Autodesk Inventor part; units mm, degrees
ref_plane "YZ Plane" through (0, 0, 0) normal (1, 0, 0) x (0, 1, 0)
ref_plane "XZ Plane" through (0, 0, 0) normal (0, 1, 0) x (-1, 0, 0)
ref_plane "XY Plane" through (0, 0, 0) normal (0, 0, 1) x (1, 0, 0)
sketch "Skizze1" plane through (0, 0, 0) normal (0, 0, 1) x (1, 0, 0)
  line L0 (-3.2332, 0) -> (3.2332, 0) construction
  line L1 (0, -2.8) -> (0, 2.8) construction
  circle A0 centre (0, 0) radius 2 construction
  line L2 (1.1547, 2) -> (2.3094, 0)
  line L3 (2.3094, 0) -> (1.1547, -2)
  line L4 (1.1547, -2) -> (-1.1547, -2)
  line L5 (-1.1547, -2) -> (-2.3094, 0)
  line L6 (-2.3094, 0) -> (-1.1547, 2)
  line L7 (-1.1547, 2) -> (1.1547, 2)
  circle A1 centre (0, 0) radius 1
  point P0 (0, 2)
  dimension "d0" = 4
  dimension "d1" = 2
extrude "Extrusion1" add sketch "Skizze1" along normal blind 20
sketch "Skizze2" plane through (0, 0, 0) normal (0, 1, 0) x (-1, 0, 0)
  line L0 (1.1547, 20) -> (-1.1547, 20)
  line L1 (-1.1547, 20) -> (-2.3094, 20)
  line L2 (2.3094, 20) -> (1.1547, 20)
  line L3 (2.3094, 0) -> (1.1547, 0)
  line L4 (1.1547, 0) -> (-1.1547, 0)
  line L5 (-1.1547, 0) -> (-2.3094, 0)
  line L6 (-1.8094, 20) -> (-3.6188, 20)
  line L7 (-3.6188, 20) -> (-3.6188, 19.3414)
  line L8 (-3.6188, 19.3414) -> (-1.8094, 20)
  line L9 (-1.8094, 0) -> (-3.6188, 0.6586)
  line L10 (-3.6188, 0.6586) -> (-3.6188, 0)
  line L11 (-3.6188, 0) -> (-1.8094, 0)
  line L12 (0, -2) -> (0, 12)
  point P0 (0, 0)
  dimension "d4" = 20
  dimension "d5" = 0.5
revolve "Umdrehung1" cut sketch "Skizze2" angle 360 about axis through (0, 0, -10) along (0, 0, 1)
properties part number "Hex Spacer 20mm"
Build history of the part. All positions in model axes, mm. Round coordinates to 2 decimals unless told otherwise and drop trailing zeros. Write each loop counter-clockwise with the first axis right and the second up, starting at its lowest first coordinate (ties: lowest second). Pieces come first, ordered by that corner, then holes.
1) Band-saw the part on B-B, the plane z = 19. List the corners of the cut face in (x, y), and give its area (3 significant figures).
2) Band-saw the part on A-A, the plane x = 0. List the corners of the cut face in (y, z), and give its area (3 significant figures).
3) Mould opens along Y. For faces 1 (the flat face through (0, 2, 10)), 2 (the flat face through (1, -1, 20)), 3 (the flat face through (0, -2, 10)), 4 (the cylindrical face through (0, 1, 10)) say: +Y half, -Y half, draft (parallel to the pull), parting line (faces both ways), or undercut.
4) Drill centre lines: probe 1 along Y at (x, z) = (0, 10.5); probe 2 along X at (y, z) = (0.2, 12); probe 3 along Y at (x, z) = (-0.7, 4.5). Where is each one in solid material? Low to high.
Ans:
1. outline: (-2.31, 0) - (-1.15, -2) - (1.15, -2) - (2.31, 0) - (1.15, 2) - (-1.15, 2) - close; hole circle Ø2 at (0, 0)
1. area: 10.7 mm2
2. outline: (-2, 0.07) - (-1.81, 0) - (-1, 0) - (-1, 20) - (-1.81, 20) - (-2, 19.93) - close; (1, 0) - (1.81, 0) - (2, 0.07) - (2, 19.93) - (1.81, 20) - (1, 20) - close
2. area: 40.0 mm2
3. face 1: +Y half
3. face 2: draft
3. face 3: -Y half
3. face 4: undercut
4. probe 1: y = -2 to -1, 1 to 2
4. probe 2: x = -2.19 to -0.98, 0.98 to 2.19
4. probe 3: y = -2 to -0.71, 0.71 to 2
